Check sheet for the modelled part. Datum: model origin and axes. Units: mm. Round coordinates to 2 decimals unless told otherwise and drop trailing zeros. Write each loop counter-clockwise with the first axis right and the second up, starting at its lowest first coordinate (ties: lowest second). Pieces come first, ordered by that corner, then holes.
Item 1: Section check D-D, the plane y = 3.75. Record the cut outline in (x, z).
Item 2: Section check A-A, the plane x = 0. Record the cut outline in (y, z), plus the area to 4 significant figures.
Item 3: Release check for a two-part mould opening along Z. For faces 1 (the flat face through (-113, -9.5, -115)), 2 (the cylindrical face through (-117.133, 0.133, -152.761)), 3 (the cylindrical face through (179.957, -0.133, -0.651)) record: pulls with the +Z half, pulls with the -Z half, needs draft (parallel to the pull), parting line crosses it, or undercut.
Item 4: Material ranges on line 1 along X through (y, z) = (2.75, 0); line 2 along Z through (x, y) = (-91, -3.5); line 3 along X through (y, z) = (5, 33), recorded low to high.
Item 5: Section check C-C, the plane x = -87.5. Record the cut outline in (y, z).
Item 6: Section check B-B, the plane z = 90.5. Record the cut outline in (x, y).
Item 7: Depth check by flat-ended pin: pin 1 (1.5 mm diameter, centred on y = -4.5, z = -25.5, fed in from -X); pin 2 (3 mm diameter, centred on y = 2, z = -51, fed in from +X); pin 3 (1 mm diameter, centred on x = 41.5, y = -6, fed in from +Z). Enter the tip coordinate at first touch or a pass-through.
from build123d import *

# Parameters (mm, degrees)
SKETCH1_R           = 192.5
SKETCH1_R_2         = 160
SKETCH1_R_3         = 5
BOSS_EXTRUDE1_DEPTH = 9.5


with BuildPart() as part:
    # Sketch1 → Boss-Extrude1 (new, symmetric)
    with BuildSketch(Plane(origin=(0, 0, 0), x_dir=(1, 0, 0), z_dir=(0, 1, 0))):
        with Locations(Location((0, 0, 0), (0, 0, 270))):
            Circle(SKETCH1_R)
        with Locations(Location((0, 0, 0), (0, 0, 270))):
            Circle(SKETCH1_R_2, mode=Mode.SUBTRACT)
        with Locations(Location((-87.5, 151.554445662, 0), (0, 0, 270))):
            Circle(SKETCH1_R_3, mode=Mode.SUBTRACT)
        with Locations(Location((-175, 0, 0), (0, 0, 270))):
            Circle(SKETCH1_R_3, mode=Mode.SUBTRACT)
        with Locations(Location((87.5, 151.554445662, 0), (0, 0, 270))):
            Circle(SKETCH1_R_3, mode=Mode.SUBTRACT)
        with Locations(Location((175, 0, 0), (0, 0, 270))):
            Circle(SKETCH1_R_3, mode=Mode.SUBTRACT)
        with Locations(Location((87.5, -151.554445662, 0), (0, 0, 90))):
            Circle(SKETCH1_R_3, mode=Mode.SUBTRACT)
        with Locations(Location((-87.5, -151.554445662, 0), (0, 0, 90))):
            Circle(SKETCH1_R_3, mode=Mode.SUBTRACT)
    extrude(amount=BOSS_EXTRUDE1_DEPTH, both=True)


solid = part.part
Values found:
1. outline: circle Ø385 at (0, 0); hole circle Ø10 at (-175, 0); hole circle Ø320 at (0, 0); hole circle Ø10 at (-87.5, -151.55); hole circle Ø10 at (-87.5, 151.55); hole circle Ø10 at (87.5, -151.55); hole circle Ø10 at (87.5, 151.55); hole circle Ø10 at (175, 0)
2. outline: (-9.5, -192.5) - (9.5, -192.5) - (9.5, -160) - (-9.5, -160) - close; (-9.5, 160) - (9.5, 160) - (9.5, 192.5) - (-9.5, 192.5) - close
2. area: 1,235 mm2
3. face 1: needs draft
3. face 2: parting line crosses it
3. face 3: undercut
4. line 1: x = -192.5 to -180, -170 to -160, 160 to 170, 180 to 192.5
4. line 2: z = -169.63 to -155.13, -147.98 to -131.6, 131.6 to 147.98, 155.13 to 169.63
4. line 3: x = -189.65 to -156.56, 156.56 to 189.65
5. outline: (-9.5, -171.46) - (9.5, -171.46) - (9.5, -156.55) - (-9.5, -156.55) - close; (-9.5, -146.55) - (9.5, -146.55) - (9.5, -133.95) - (-9.5, -133.95) - close; (-9.5, 133.95) - (9.5, 133.95) - (9.5, 146.55) - (-9.5, 146.55) - close; (-9.5, 156.55) - (9.5, 156.55) - (9.5, 171.46) - (-9.5, 171.46) - close
6. outline: (-169.9, -9.5) - (-131.95, -9.5) - (-131.95, 9.5) - (-169.9, 9.5) - close; (131.95, -9.5) - (169.9, -9.5) - (169.9, 9.5) - (131.95, 9.5) - close
7. pin 1: stops at x = -190.9
7. pin 2: stops at x = 186.03
7. pin 3: stops at z = 188.08
